Source: CAD feature listing. Evaluate the final solid. Frame: model axes, mm. A direction names the side the tool comes from. Round coordinates to 2 decimals unless told otherwise and drop trailing zeros. Order: outer loops, then holes, each group sorted by start corner. A loop starts at its lowest first (then second) coordinate and runs counter-clockwise, first axis right, second up. Notation, with made-up numbers: (76.5, -7.75) - (120.5, -7.75) arc R10 cw to (120.5, 8.25) - close; hole circle Ø1 at (0.5, 47). An arc over 180 degrees is marked (long way). Put each result on its own line as item: value. Start each with the question number.
1) Section C-C on z = 6. Output: boundary loops of the cut face in (x, y).
2) Section B-B on y = -19. Output: boundary loops of the cut face in (x, z), then the cut area to 3 significant figures.
3) Contact query for flat-ended pins moving along their axis: P1, Ø6.5, axis at x = 8.25, z = 6, coming from the -Y side; P2, Ø6, axis at y = -20.5, z = 3, coming from the -X side; P3, Ø6, axis at y = -25.5, z = 7.5, coming from the +X side. Output: stop coordinate, or through.
4) Mould query, pull axis X, two halves, no side actions, for faces 4 (the face through (-54, -22, 6)), 5 (the face through (-52, -19, 6)), 6 (the face through (-60, 0, 3)), 7 (the face through (-57.865, 1.479, 6.751)). Classes: +X half, -X half, draft (parallel to the pull), parting line (faces both ways), or undercut.
5) Section D-D on z = 10.25. Output: boundary loops of the cut face in (x, y), then the cut area to 3 significant figures.
6) Access query for faces 1 (the face through (-26, -42, 6)), 2 (the face through (-26, -43, 12)), 3 (the face through (8, 0, 9)). Directions: +Z, -Z, +X, -X, +Y, -Y. A direction counts if a zero-diameter tool reaches every point of the face in a straight line with its end or side. Return the directions, or none.
7) Section A-A on x = 8.25. Output: boundary loops of the cut face in (y, z), then the cut area to 3 significant figures.
8) Line query: probe 1 along X at (y, z) = (-12, 8.75); probe 2 along Z at (x, y) = (-60, 1); probe 3 along Y at (x, z) = (-45, 4). Output: solid intervals per line, ascending. Write a range as [from, to].
```python
from build123d import *

# Parameters (mm, degrees)
BOSS_EXTRUDE1_DEPTH = 12
SKETCH3_W           = 12
SKETCH3_H           = 3
BOSS_EXTRUDE2_DEPTH = 2.5
SKETCH4_W           = 12
SKETCH4_H           = 3
BOSS_EXTRUDE3_DEPTH = 2.5
SKETCH6_R           = 2.5
CUT_EXTRUDE1_DEPTH  = 10
SKETCH7_R           = 2.5
CUT_EXTRUDE2_DEPTH  = 10


with BuildPart() as part:
    # Sketch1 → Boss-Extrude1 (new body)
    with BuildSketch(Plane.XY):
        Polygon((0, 0), (0, 3), (12, 3), (12, 0), (2, 0), (2, -44), (-54, -44), (-54, 0), (-64, 0), (-64, 3), (-52, 3), (-52, -42), (0, -42), align=None)
    extrude(amount=BOSS_EXTRUDE1_DEPTH)

    # Sketch3 → Boss-Extrude2 (add)
    with BuildSketch(Plane(origin=(12, 0, 0), x_dir=(0, 0, -1), z_dir=(1, 0, 0))):
        with Locations((-6, 1.5)):
            Rectangle(SKETCH3_W, SKETCH3_H)
    extrude(amount=BOSS_EXTRUDE2_DEPTH)

    # Sketch4 → Boss-Extrude3 (add)
    with BuildSketch(Plane.ZY.offset(64)):
        with Locations((6, 1.5)):
            Rectangle(SKETCH4_W, SKETCH4_H)
    extrude(amount=BOSS_EXTRUDE3_DEPTH)

    # Sketch6 → Cut-Extrude1 (cut)
    with BuildSketch(Plane.XZ):
        with Locations((-60.25, 6)):
            Circle(SKETCH6_R)
    extrude(amount=-CUT_EXTRUDE1_DEPTH, mode=Mode.SUBTRACT)

    # Sketch7 → Cut-Extrude2 (cut)
    with BuildSketch(Plane.XZ):
        with Locations((8.25, 6)):
            Circle(SKETCH7_R)
    extrude(amount=-CUT_EXTRUDE2_DEPTH, mode=Mode.SUBTRACT)


solid = part.part
```
Answer sheet:
1. outline: (-66.5, 0) - (-62.75, 0) - (-62.75, 3) - (-66.5, 3) - close; (-57.75, 0) - (-54, 0) - (-54, -44) - (2, -44) - (2, 0) - (5.75, 0) - (5.75, 3) - (0, 3) - (0, -42) - (-52, -42) - (-52, 3) - (-57.75, 3) - close; (10.75, 0) - (14.5, 0) - (14.5, 3) - (10.75, 3) - close
2. outline: (-54, 0) - (-52, 0) - (-52, 12) - (-54, 12) - close; (0, 0) - (2, 0) - (2, 12) - (0, 12) - close
2. area: 48.0 mm^2
3. P1: y = 0
3. P2: x = -54
3. P3: x = 2
4. face 4: -X half
4. face 5: undercut
4. face 6: draft
4. face 7: undercut
5. outline: (-66.5, 0) - (-54, 0) - (-54, -44) - (2, -44) - (2, 0) - (14.5, 0) - (14.5, 3) - (0, 3) - (0, -42) - (-52, -42) - (-52, 3) - (-66.5, 3) - close
5. area: 367 mm^2
6. face 1: +Z, -Z, +Y
6. face 2: +Z, +X, -X, +Y, -Y
6. face 3: +Z, -Z, +X, -Y
7. outline: (0, 0) - (3, 0) - (3, 3.5) - (0, 3.5) - close; (0, 8.5) - (3, 8.5) - (3, 12) - (0, 12) - close
7. area: 21.0 mm^2
8. probe 1: [-54, -52], [0, 2]
8. probe 2: [0, 3.51], [8.49, 12]
8. probe 3: [-44, -42]
